from build123d import *

# Parameters (mm, degrees)
SKETCH_1_W          = 43
SKETCH_1_H          = 43
SKETCH_1_R          = 1.75
SKETCH_1_R_2        = 12.5
EXTRUDE_1_DEPTH     = 5
SKETCH_3_W          = 43
SKETCH_3_H          = 5
EXTRUDE_2_DEPTH     = 5
SKETCH_4_W          = 43
SKETCH_4_H          = 50
EXTRUDE_3_DEPTH     = 5
SKETCH_5_R          = 2.75
CUT_EXTRUDE_1_DEPTH = 79.056311978
SKETCH_6_W          = 43
SKETCH_6_H          = 5
EXTRUDE_4_DEPTH     = 15
CUT_EXTRUDE_2_DEPTH = 72.979728546


with BuildPart() as part:
    # 草图1 → 凸台-拉伸1 (new body)
    with BuildSketch(Plane(origin=(0, 0, 0), x_dir=(1, 0, 0), z_dir=(0, 1, 0))):
        with Locations((-14.399691358, 11.712191358)):
            Rectangle(SKETCH_1_W, SKETCH_1_H)
        with Locations(Location((1.100308642, 27.212191358, 0), (0, 0, 270))):
            Circle(SKETCH_1_R, mode=Mode.SUBTRACT)
        with Locations(Location((-29.899691358, 27.212191358, 0), (0, 0, 270))):
            Circle(SKETCH_1_R, mode=Mode.SUBTRACT)
        with Locations(Location((-29.899691358, -3.787808642, 0), (0, 0, 270))):
            Circle(SKETCH_1_R, mode=Mode.SUBTRACT)
        with Locations(Location((1.100308642, -3.787808642, 0), (0, 0, 270))):
            Circle(SKETCH_1_R, mode=Mode.SUBTRACT)
        with Locations(Location((-14.399691358, 11.712191358, 0), (0, 0, 270))):
            Circle(SKETCH_1_R_2, mode=Mode.SUBTRACT)
    extrude(amount=EXTRUDE_1_DEPTH)

    # 草图3 → 凸台-拉伸2 (add)
    with BuildSketch(Plane(origin=(0, 0, -33.212191358), x_dir=(-1, 0, 0), z_dir=(0, 0, -1))):
        with Locations((14.399691358, 2.5)):
            Rectangle(SKETCH_3_W, SKETCH_3_H)
    extrude(amount=EXTRUDE_2_DEPTH)

    # 草图4 → 凸台-拉伸3 (add)
    with BuildSketch(Plane(origin=(0, 0, -38.212191358), x_dir=(-1, 0, 0), z_dir=(0, 0, -1))):
        with Locations((14.399691358, 25)):
            Rectangle(SKETCH_4_W, SKETCH_4_H)
    extrude(amount=EXTRUDE_3_DEPTH)

    # 草图5 → 切除-拉伸1 (cut, through all)
    with BuildSketch(Plane.XY.offset(-38.212191358)):
        with Locations((-14.399691358, 43)):
            Circle(SKETCH_5_R)
        with Locations((-14.399691358, 12)):
            Circle(SKETCH_5_R)
    extrude(amount=-CUT_EXTRUDE_1_DEPTH, mode=Mode.SUBTRACT)

    # 草图6 → 凸台-拉伸4 (add)
    with BuildSketch(Plane.XY.offset(9.787808642)):
        with Locations((-14.399691358, 2.5)):
            Rectangle(SKETCH_6_W, SKETCH_6_H)
    extrude(amount=EXTRUDE_4_DEPTH)

    # 草图7 → 切除-拉伸2 (cut, through all)
    with BuildSketch(Plane(origin=(0, 5, 0), x_dir=(1, 0, 0), z_dir=(0, 1, 0))):
        with BuildLine():
            Line((-17.899691358, -18.037808642), (-7.899691358, -18.037808642))
            ThreePointArc((-7.899691358, -18.037808642), (-6.149691358, -19.787808642), (-7.899691358, -21.537808642))
            Line((-7.899691358, -21.537808642), (-17.899691358, -21.537808642))
            ThreePointArc((-17.899691358, -21.537808642), (-19.649691358, -19.787808642), (-17.899691358, -18.037808642))
        make_face()
    extrude(amount=-CUT_EXTRUDE_2_DEPTH, mode=Mode.SUBTRACT)


solid = part.part
Geometry check sheet. Reference: the model listing, model coordinates, mm. A direction names the side the tool comes from. Give positions to 0.01 mm unless a question says otherwise; leave off trailing zeros. Loops run counter-clockwise (first coordinate to the right, second up) from the corner with the lowest first, then second, coordinate; pieces in that order, holes last. Notation, with made-up numbers: M -10.5,59 L 40.5,59 A35 ccw 40.5,95 Z; hole C 66.25,68 d5. An arc over 180 degrees is marked long. Answer as a JSON object with one key per item and string values. Group by question number.
Item 1: Sectioned sample at B-B on x = -13. Record the boundary of the cut face in (y, z).
Item 2: Sectioned sample at C-C on z = -10. Record the boundary of the cut face in (x, y), plus the area to 3 significant figures.
Item 3: Sectioned sample at D-D on y = 23. Record the boundary of the cut face in (x, z), plus the area to 3 significant figures.
Item 4: Access from +Z, -Z, +X, -X, +Y, -Y to the whole of each face (thin tool, end or side, straight path). Record for faces 1 (the flat face through (-14, 28, -38.212)), 2 (the cylindrical face through (-16.427, 13.859, -40.677)), 3 (the cylindrical face through (-6.15, 2.54, 19.75)).
Item 5: Mould release check, pull along X, two halves, no side actions. Record for faces 4 (the cylindrical face through (1.18, 2.46, -28.96)), 5 (the flat face through (7.1, 4.5, -19.4)), 6 (the flat face through (-24, 5, 0)): pulls with the +X half, pulls with the -X half, needs draft (parallel to the pull), parting line crosses it, or undercut.
Item 6: Material ranges on L1, parallel to Z at x = 3, y = 24; L2, parallel to Y at x = -32, z = 17, recorded low to high.
Item 7: Sectioned sample at A-A on y = 43. Record the boundary of the cut face in (x, z), plus the area to 4 significant figures.
Item 8: Gauge pin test, flat ends, axial feed: pin 1 (12 mm diameter, centred on x = -1.5, z = 14.5, fed in from -Y); pin 2 (3 mm diameter, centred on x = -22.5, y = 14.5, fed in from +Z); pin 3 (4.5 mm diameter, centred on x = 1.1, z = -27.21, fed in from +Y). Record the tip position at first contact, or that the pin passes through.
Findings below:
{
 "1": {"outline": "M 0,-43.21 L 9.63,-43.21 L 9.63,-38.21 L 5,-38.21 L 5,-24.13 L 0,-24.13 Z; M 0,0.71 L 5,0.71 L 5,18.04 L 0,18.04 Z; M 0,21.54 L 5,21.54 L 5,24.79 L 0,24.79 Z; M 14.37,-43.21 L 40.63,-43.21 L 40.63,-38.21 L 14.37,-38.21 Z; M 45.37,-43.21 L 50,-43.21 L 50,-38.21 L 45.37,-38.21 Z"},
 "2": {"outline": "M -35.9,0 L -26.78,0 L -26.78,5 L -35.9,5 Z; M -2.02,0 L 7.1,0 L 7.1,5 L -2.02,5 Z", "area": "91.2 mm2"},
 "3": {"outline": "M -35.9,-43.21 L 7.1,-43.21 L 7.1,-38.21 L -35.9,-38.21 Z", "area": "215 mm2"},
 "4": {"face 1": "+Z, +X, -X, +Y", "face 2": "+Z, -Z", "face 3": "+Y, -Y"},
 "5": {"face 4": "undercut", "face 5": "pulls with the +X half", "face 6": "needs draft"},
 "6": {"L1": "-43.21 to -38.21", "L2": "0 to 5"},
 "7": {"outline": "M -35.9,-43.21 L -17.15,-43.21 L -17.15,-38.21 L -35.9,-38.21 Z; M -11.65,-43.21 L 7.1,-43.21 L 7.1,-38.21 L -11.65,-38.21 Z", "area": "187.5 mm2"},
 "8": {"pin 1": "y = 0", "pin 2": "z = -38.21", "pin 3": "y = 5"}
}
